Geometry: final body of the model. Coordinates: model frame, mm. A direction names the side the tool comes from. Give positions to 0.01 mm unless a question says otherwise; leave off trailing zeros. Order: outer loops, then holes, each group sorted by start corner. A loop starts at its lowest first (then second) coordinate and runs counter-clockwise, first axis right, second up. Notation, with made-up numbers: (-9, -12) - (-5, -12) arc R14 cw to (-5, -1) - close; hole circle Ø11 at (71, -21). An arc over 180 degrees is marked (long way). Put each result on its own line as item: value. Start each with the question number.
1. First-contact query: P1, Ø2.5, axis at x = 2.5, y = 22, coming from the +Z side; P2, Ø1, axis at x = 2.5, z = -23.5, coming from the +Y side; P3, Ø6.5, axis at y = 60, z = 1, coming from the -X side; P4, Ø2.5, axis at y = 24, z = -32, coming from the +X side. Flat tips, straight axial feed; report the tip coordinate or a pass-through.
2. Section C-C on x = 2.9. Count the separate pieces of the cut face and the enclosed holes in it, plus the area to 3 significant figures.
3. Section B-B on y = 24. Return the cut outline in (x, z).
4. Mould query, pull axis Y, two halves, no side actions, for faces 1 (the cylindrical face through (2.465, 56.17, -29.237)), 2 (the flat face through (2, 20, -40)), 3 (the flat face through (2.465, 46.41, 1.974)). Classes: pulls with the +Y half, pulls with the -Y half, needs draft (parallel to the pull), parting line crosses it, or undercut.
5. Ray query, line 1 along Y through (x, z) = (1.7, -20); line 2 along Y through (x, z) = (3.85, -32); line 3 along Y through (x, z) = (3, -7.5). Return the intervals inside material, ascending. Write a range as from..to.
6. Section D-D on y = 39. Return the cut outline in (x, z).
7. Section A-A on z = -20. Return the cut outline in (x, y), plus the area to 3 significant figures.
8. Set-up query: faces 4 (the flat face through (2, 20, 0)), 5 (the cylindrical face through (2.465, 12.601, -33.908)). Return all of +Z, -Z, +X, -X, +Y, -Y with unobstructed straight access to the full face (end or side cutting, diameter ignored); none if empty.
from build123d import *

# Parameters (mm, degrees)
CROQUIS1_R              = 2
CROQUIS1_R_2            = 2.5
CROQUIS1_R_3            = 10
SALIENTE_EXTRUIR1_DEPTH = 5


with BuildPart() as part:
    # Croquis1 → Saliente-Extruir1 (new body)
    with BuildSketch(Plane(origin=(0, 0, 0), x_dir=(0, 0, -1), z_dir=(1, 0, 0))):
        with BuildLine():
            ThreePointArc((43.892972847, 52.642972847), (20, 85), (-3.892972847, 52.642972847))
            Line((-3.892972847, 52.642972847), (0, 40))
            Line((0, 40), (0, 0))
            Line((0, 0), (40, 0))
            Line((40, 0), (40, 40))
            Line((40, 40), (43.892972847, 52.642972847))
        make_face()
        with Locations((8, 12)):
            Circle(CROQUIS1_R, mode=Mode.SUBTRACT)
        with Locations((8, 24)):
            Circle(CROQUIS1_R, mode=Mode.SUBTRACT)
        with Locations((20, 39)):
            Circle(CROQUIS1_R_2, mode=Mode.SUBTRACT)
        with Locations((32, 12)):
            Circle(CROQUIS1_R, mode=Mode.SUBTRACT)
        with Locations((32, 24)):
            Circle(CROQUIS1_R, mode=Mode.SUBTRACT)
        with Locations((-1, 60)):
            Circle(CROQUIS1_R_2, mode=Mode.SUBTRACT)
        with Locations((20, 60)):
            Circle(CROQUIS1_R_3, mode=Mode.SUBTRACT)
        with Locations((20, 81)):
            Circle(CROQUIS1_R_2, mode=Mode.SUBTRACT)
        with Locations((41, 60)):
            Circle(CROQUIS1_R_2, mode=Mode.SUBTRACT)
    extrude(amount=SALIENTE_EXTRUIR1_DEPTH)


solid = part.part
Resolved:
1. P1: z = 0
1. P2: y = 84.82
1. P3: x = 0
1. P4: through
2. separate pieces: 1
2. enclosed holes: 9
2. area: 3,060 mm^2
3. outline: (0, -40) - (5, -40) - (5, -34) - (0, -34) - close; (0, -30) - (5, -30) - (5, -10) - (0, -10) - close; (0, -6) - (5, -6) - (5, 0) - (0, 0) - close
4. face 1: undercut
4. face 2: needs draft
4. face 3: pulls with the -Y half
5. line 1: 0..36.5, 41.5..50, 70..78.5, 83.5..85
5. line 2: 0..10, 14..22, 26..81.93
5. line 3: 0..10.06, 13.94..22.06, 25.94..81.65
6. outline: (0, -40) - (5, -40) - (5, -22.5) - (0, -22.5) - close; (0, -17.5) - (5, -17.5) - (5, 0) - (0, 0) - close
7. outline: (0, 0) - (5, 0) - (5, 36.5) - (0, 36.5) - close; (0, 41.5) - (5, 41.5) - (5, 50) - (0, 50) - close; (0, 70) - (5, 70) - (5, 78.5) - (0, 78.5) - close; (0, 83.5) - (5, 83.5) - (5, 85) - (0, 85) - close
7. area: 275 mm^2
8. face 4: +Z, +X, -X, -Y
8. face 5: +X, -X
